from build123d import *

# Parameters (mm, degrees)
CYLINDER043_R          = 1.7
CYLINDER043_DEPTH      = 10
CYLINDER043_ROLL_ANGLE = 90
CYLINDER044_R          = 1.7
CYLINDER044_DEPTH      = 10
CYLINDER044_ROLL_ANGLE = 90
BOX080_W               = 44
BOX080_H               = 2
BOX080_DEPTH           = 31


with BuildPart() as cylinder075:
    # Cylinder043 → Cylinder043 (new body)
    with BuildSketch(Plane.XY):
        Circle(CYLINDER043_R)
    extrude(amount=CYLINDER043_DEPTH)


with BuildPart() as cylinder075_1:
    # Cylinder043 roll: moved
    add(cylinder075.part.rotate(Axis((0, 0, 0), (1, 0, 0)), CYLINDER043_ROLL_ANGLE))


with BuildPart() as cylinder075_2:
    # Cylinder043 placement: moved
    add(cylinder075_1.part.moved(Location((26, 70, 20))))


with BuildPart() as cylinder076:
    # Cylinder044 → Cylinder044 (new body)
    with BuildSketch(Plane.XY):
        Circle(CYLINDER044_R)
    extrude(amount=CYLINDER044_DEPTH)


with BuildPart() as cylinder076_1:
    # Cylinder044 roll: moved
    add(cylinder076.part.rotate(Axis((0, 0, 0), (1, 0, 0)), CYLINDER044_ROLL_ANGLE))


with BuildPart() as cylinder076_2:
    # Cylinder044 placement: moved
    add(cylinder076_1.part.moved(Location((65, 70, 20))))


with BuildPart() as obj1:
    # Box080 → Box080 (new body)
    with BuildSketch(Plane(origin=(23.5, 68, 4.5), x_dir=(1, 0, 0), z_dir=(0, 0, 1))):
        with Locations((22, 1)):
            Rectangle(BOX080_W, BOX080_H)
    extrude(amount=BOX080_DEPTH)

    # Cut090: cut Cylinder076
    add(cylinder076_2.part, mode=Mode.SUBTRACT)

    # Cut091: cut Cylinder075
    add(cylinder075_2.part, mode=Mode.SUBTRACT)


solid = obj1.part
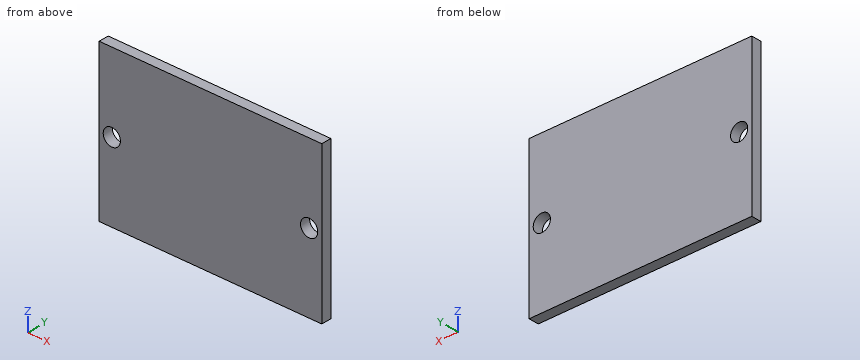
The listing builds one solid part. Answer for the finished solid, in the listing's coordinates (mm). Coordinates: 2 decimals unless noted, no trailing zeros. Order: outer loops, then holes, each group sorted by start corner. A loop starts at its lowest first (then second) coordinate and runs counter-clockwise, first axis right, second up.
Q1. A cutting plane is placed at B-B, the plane x = 65. Write down the section's boundary in (y, z).
Q2. Consider line 1 (X direction, y = 69.6, z = 20); line 2 (Z direction, x = 65, y = 68.55); line 3 (X direction, y = 69.85, z = 20.5). Determine where each line is inside the solid, lowest interval first.
Q3. A cutting plane is placed at A-A, the plane z = 20. Write down the section's boundary in (x, y).
Answers follow:
1. outline: (68, 4.5) - (70, 4.5) - (70, 18.3) - (68, 18.3) - close; (68, 21.7) - (70, 21.7) - (70, 35.5) - (68, 35.5) - close
2. line 1: x = 23.5 to 24.3, 27.7 to 63.3, 66.7 to 67.5
2. line 2: z = 4.5 to 18.3, 21.7 to 35.5
2. line 3: x = 23.5 to 24.38, 27.62 to 63.38, 66.62 to 67.5
3. outline: (23.5, 68) - (24.3, 68) - (24.3, 70) - (23.5, 70) - close; (27.7, 68) - (63.3, 68) - (63.3, 70) - (27.7, 70) - close; (66.7, 68) - (67.5, 68) - (67.5, 70) - (66.7, 70) - close
